from build123d import *

# Parameters (mm, degrees)
F1_DEPTH      = 6.35
F3_ANGLE_BACK = 8
F3_ANGLE      = 16


with BuildPart() as f1:
    # F0 (on Top) → F1 (new body)
    with BuildSketch(Plane.XY):
        with BuildLine():
            ThreePointArc((-10.16, 69.1071407309), (-5.093560638, 69.664037638), (0, 69.85))
            ThreePointArc((0, 69.85), (5.0595865172, 69.6665133638), (10.0925913162, 69.1170174452))
            Line((10.0925913162, 69.1170174452), (10.0925913162, 88.1571407309))
            Line((10.0925913162, 88.1571407309), (-10.16, 88.1571407309))
            Line((-10.16, 88.1571407309), (-10.16, 69.1071407309))
        make_face()
        with BuildLine():
            ThreePointArc((10.0925913162, 69.1170174452), (5.0595865172, 69.6665133638), (0, 69.85))
            ThreePointArc((0, 69.85), (-5.093560638, 69.664037638), (-10.16, 69.1071407309))
            Line((-10.16, 69.1071407309), (-10.16, 47.625))
            ThreePointArc((-10.16, 47.625), (-0.5851804113, 37.4818661704), (10.0925913162, 46.456582042))
            Line((10.0925913162, 46.456582042), (10.0925913162, 69.1071407309))
            Line((10.0925913162, 69.1071407309), (10.0925913162, 69.1170174452))
        make_face()
        with BuildLine():
            ThreePointArc((3.556, 47.625), (-2.5144717139, 45.1105282861), (0, 51.181))
            ThreePointArc((0, 51.181), (2.5144717139, 50.1394717139), (3.556, 47.625))
        make_face(mode=Mode.SUBTRACT)
    extrude(amount=F1_DEPTH)

    # F2 (on Right) → F3 (revolve)
    with BuildSketch(Plane.YZ, mode=Mode.PRIVATE) as f3_sk:
        Polygon((69.85, 6.35), (69.85, 0), (109.1197147274, 0), (109.8804209793, 2.8389943816), (73.0786469976, 12.7), (69.85, 12.7), align=None)
    revolve(f3_sk.sketch.rotate(Axis((0, 0, 0), (0, 0, 1)), -F3_ANGLE_BACK), axis=Axis((0, 0, 0), (0, 0, 1)), revolution_arc=F3_ANGLE)

    # F4 (on Right) → F5 (revolve, cut)
    with BuildSketch(Plane.YZ):
        Polygon((91.6529184641, 9.2004434954), (90.8311679959, 6.1336289969), (109.2320549867, 1.2031261877), (110.0538054549, 4.2699406862), align=None)
    revolve(axis=Axis((0, 91.24204323, 7.6670362462), (0, 0.2588190451, 0.9659258263)), mode=Mode.SUBTRACT)


solid = f1.part
Could you check a few things on this model? Use its own coordinates, in mm. A direction names the side the tool comes from. Round coordinates to 2 decimals unless told otherwise and drop trailing zeros. Write each loop counter-clockwise with the first axis right and the second up, starting at its lowest first coordinate (ties: lowest second). Pieces come first, ordered by that corner, then holes. Notation, with made-up numbers: (12, 73) - (26, 73) arc R26 cw to (26, 107) - close; hole circle Ø1 at (86, 65). An arc over 180 degrees is marked (long way). Put each result on its own line as item: value. Start each with the question number.
(1) I want a section at C-C, the plane z = 8.5. Please give me the cut outline in (x, y).
(2) Will these pins go through, and if not, where does the flat tip stop? pin 1 (12 mm diameter, centred on x = 0, y = 48, fed in from +Z); pin 2 (1.5 mm diameter, centred on x = -7.5, y = 78, fed in from +Z); pin 3 (4 mm diameter, centred on x = 11, y = 98, fed in from +Z); pin 4 (6 mm diameter, centred on y = 51.5, z = 10, fed in from +X).
(3) I want a section at B-B, the plane y = 59.5. Please give me the cut outline in (x, z).
(4) For faces 1 (the cylindrical face through (0.14, 69.85, 9.48)), 2 (the conical face through (4.6, 109.45, 2.93)), 3 (the cylindrical face through (-0.159, 72.659, 11.915)), 4 (the flat face through (10.093, 59, 3)), 5 (the flat face through (-10.16, 60, 3)), which set-ups out of +Z, -Z, +X, -X, +Y, -Y let a thin tool reach every point of the face, with its end or its side?
(5) Thinking about a two-plate mould opening in Y: for faces 6 (the flat face through (0, 55, 6.35)), 7 (the cylindrical face through (-0.8, 37.497, 3.131)), 8 (the cylindrical face through (0.23, 109.46, 2.06)), 9 (the cylindrical face through (1.068, 51.017, 3.131)), which applies, released by +Y, released by -Y, zero draft, split by the parting line, or undercut?
(6) I need wall thicknesses on probe 1 along Z at (x, y) = (-6, 90); probe 2 along X at (y, z) = (71, 5); probe 3 along Z at (x, y) = (-4, 76). Which ranges of each line are inside material? Lowest first, please.
Here are the results:
1. outline: (-11.52, 82) - (-9.72, 69.17) arc R69.85 cw to (9.72, 69.17) - (11.52, 82) - close
2. pin 1: stops at z = 6.35
2. pin 2: stops at z = 9.77
2. pin 3: stops at z = 4.75
2. pin 4: passes through
3. outline: (-10.16, 0) - (10.09, 0) - (10.09, 6.35) - (-10.16, 6.35) - close
4. face 1: +Z, -Y
4. face 2: +Z, +Y
4. face 3: +Y
4. face 4: +Z, -Z, +X, -Y
4. face 5: +Z, -Z, -X, -Y
5. face 6: zero draft
5. face 7: released by -Y
5. face 8: undercut
5. face 9: undercut
6. probe 1: z = 0 to 6.36
6. probe 2: x = -10.16 to 10.09
6. probe 3: z = 0 to 10.11
